```python
from build123d import *

# Parameters (mm, degrees)
SKETCH_R        = 1.6
PAD_DEPTH       = 15
POCKET_DEPTH    = 3.5
POCKET001_DEPTH = 2.5
POCKET002_DEPTH = 2.5


with BuildPart() as part:
    # Sketch → Pad (new body)
    with BuildSketch(Plane.XY):
        with BuildLine():
            Line((-15.5, 6), (15.5, 6))
            Line((15.5, 6), (21.5, 6))
            ThreePointArc((21.5, -6), (27.5, 0), (21.5, 6))
            Line((15.5, -6), (21.5, -6))
            Line((15.5, -6), (-15.5, -6))
            Line((-15.5, -6), (-15.5, 6))
        make_face()
        with Locations((-9.5, 0)):
            Circle(SKETCH_R, mode=Mode.SUBTRACT)
        with Locations((-1.5, 0)):
            Circle(SKETCH_R, mode=Mode.SUBTRACT)
        with Locations((21.5, 0)):
            Circle(SKETCH_R, mode=Mode.SUBTRACT)
    extrude(amount=PAD_DEPTH)

    # Sketch001 (on Face11 of Pad) → Pocket (cut)
    with BuildSketch(Plane.XY.offset(15)):
        Polygon((-7.883419, 2.8), (-11.116581, 2.8), (-12.733162, 0), (-11.116581, -2.8), (-7.883419, -2.8), (-6.266838, 0), align=None)
        Polygon((0.116581, 2.8), (-3.116581, 2.8), (-4.733162, 0), (-3.116581, -2.8), (0.116581, -2.8), (1.733162, 0), align=None)
    extrude(amount=-POCKET_DEPTH, mode=Mode.SUBTRACT)

    # Sketch002 (on Face5 of Pocket) → Pocket001 (cut)
    with BuildSketch(Plane.XY.offset(15)):
        Polygon((23.116581, 2.8), (19.883419, 2.8), (18.266838, 0), (19.883419, -2.8), (23.116581, -2.8), (24.733162, 0), align=None)
    extrude(amount=-POCKET001_DEPTH, mode=Mode.SUBTRACT)

    # Sketch003 (on Face4 of Pocket001) → Pocket002 (cut)
    with BuildSketch(Plane(origin=(0, 0, 0), x_dir=(1, 0, 0), z_dir=(0, 0, -1))):
        Polygon((24.733162, 0), (23.116581, 2.8), (19.883419, 2.8), (18.266838, 0), (19.883419, -2.8), (23.116581, -2.8), align=None)
    extrude(amount=-POCKET002_DEPTH, mode=Mode.SUBTRACT)


solid = part.part
```
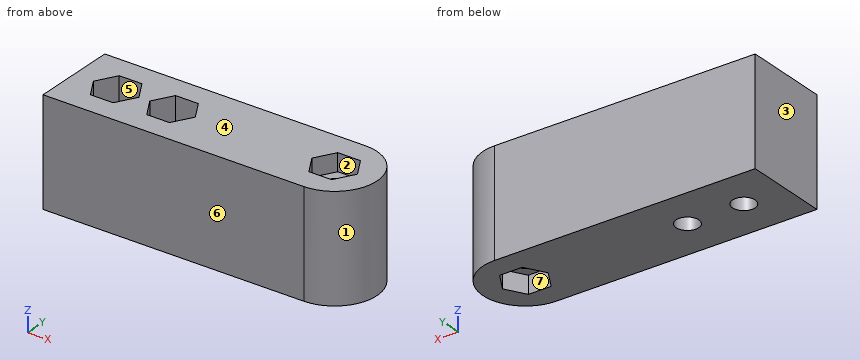
Input: part model. Units: mm. Frame: model coordinates. Face numbers are marked on the shaded views. A direction names the side the tool comes from. Give positions to 0.01 mm unless a question says otherwise; leave off trailing zeros. Order: outer loops, then holes, each group sorted by start corner. A loop starts at its lowest first (then second) coordinate and runs counter-clockwise, first axis right, second up. Notation, with made-up numbers: (26, 51.5) - (31, 51.5) arc R15 cw to (31, 79.5) - close; hole circle Ø11 at (86.25, -17). An arc over 180 degrees is marked (long way). Use a Markdown table: item, result.
(1) Access query for the marked faces 5, 6 and 7. Directions: +Z, -Z, +X, -X, +Y, -Y. A direction counts if a zero-diameter tool reaches every point of the face in a straight line with its end or side. Return the directions, or none.
Computed values:
| item | result |
|---|---|
| face 5 | +Z |
| face 6 | +Z, -Z, +X, -X, -Y |
| face 7 | -Z |
(2) Draft query along X for the marked faces 1, 2, 3 and 4. Return one class per face: released by +X, released by -X, zero draft, split by the parting line, or undercut.
Computed values:
| item | result |
|---|---|
| face 1 | released by +X |
| face 2 | undercut |
| face 3 | released by -X |
| face 4 | zero draft |
(3) Section query C-C (y = -2.25). Output: boundary loops of the cut face in (x, z).
Computed values:
| item | result |
|---|---|
| outline | (-15.5, 0) - (19.57, 0) - (19.57, 2.5) - (23.43, 2.5) - (23.43, 0) - (27.06, 0) - (27.06, 15) - (23.43, 15) - (23.43, 12.5) - (19.57, 12.5) - (19.57, 15) - (0.43, 15) - (0.43, 11.5) - (-3.43, 11.5) - (-3.43, 15) - (-7.57, 15) - (-7.57, 11.5) - (-11.43, 11.5) - (-11.43, 15) - (-15.5, 15) - close |
(4) Section query A-A (x = -1.5). Output: boundary loops of the cut face in (y, z).
Computed values:
| item | result |
|---|---|
| outline | (-6, 0) - (-1.6, 0) - (-1.6, 11.5) - (-2.8, 11.5) - (-2.8, 15) - (-6, 15) - close; (1.6, 0) - (6, 0) - (6, 15) - (2.8, 15) - (2.8, 11.5) - (1.6, 11.5) - close |
(5) Pin query (flat end, axial travel): pin 1 (5 mm diameter, centred on x = 18.5, y = -2, fed in from -Z); pin 2 (3.5 mm diameter, centred on x = 21.5, y = 0, fed in from +Z); pin 3 (3 mm diameter, centred on x = -2.5, y = -0.5, fed in from +Z); pin 4 (3 mm diameter, centred on x = -9.5, y = 0, fed in from -Z). Return the tip coordinate at first contact, or that it passes through.
Computed values:
| item | result |
|---|---|
| pin 1 | stops at z = 0 |
| pin 2 | stops at z = 12.5 |
| pin 3 | stops at z = 11.5 |
| pin 4 | passes through |
(6) Section query B-B (z = 1.75). Output: boundary loops of the cut face in (x, y), then the cut area to 3 significant figures.
Computed values:
| item | result |
|---|---|
| outline | (-15.5, -6) - (21.5, -6) arc R6 ccw to (21.5, 6) - (-15.5, 6) - close; hole circle Ø3.2 at (-9.5, 0); hole circle Ø3.2 at (-1.5, 0); hole (18.27, 0) - (19.88, -2.8) - (23.12, -2.8) - (24.73, 0) - (23.12, 2.8) - (19.88, 2.8) - close |
| area | 457 mm2 |
(7) Section query D-D (x = -7). Output: boundary loops of the cut face in (y, z), then the cut area to 3 significant figures.
Computed values:
| item | result |
|---|---|
| outline | (-6, 0) - (6, 0) - (6, 15) - (1.27, 15) - (1.27, 11.5) - (-1.27, 11.5) - (-1.27, 15) - (-6, 15) - close |
| area | 171 mm2 |
(8) Line query: line 1 (X direction, y = 0, z = 4); line 2 (X direction, y = 0, z = 13.75); line 3 (Y direction, x = -1.5, z = 7). Output: solid intervals per line, ascending. Write a range as from..to.
Computed values:
| item | result |
|---|---|
| line 1 | x = -15.5..-11.1, -7.9..-3.1, 0.1..19.9, 23.1..27.5 |
| line 2 | x = -15.5..-12.73, -6.27..-4.73, 1.73..18.27, 24.73..27.5 |
| line 3 | y = -6..-1.6, 1.6..6 |
